Can you work these out from the model? Positions are in its coordinate system, mm. Face numbers are marked on the shaded views. A direction names the side the tool comes from. Give positions to 0.01 mm unless a question says otherwise; leave off trailing zeros. Write each loop counter-clockwise with the first axis right and the second up, starting at its lowest first coordinate (ties: lowest second). Pieces come first, ordered by that corner, then holes.
```python
from build123d import *

# Parameters (mm, degrees)
SALIENTE_EXTRUIR1_DEPTH = 16
CROQUIS6_R              = 11.15
CORTAR_EXTRUIR4_DEPTH   = 14
CROQUIS22_R             = 6
CORTAR_EXTRUIR17_DEPTH  = 3
CROQUIS8_R              = 4.05
CORTAR_EXTRUIR6_DEPTH   = 17
CORTAR_EXTRUIR12_DEPTH  = 30
CROQUIS18_R             = 2.675
CORTAR_EXTRUIR13_DEPTH  = 15
CORTAR_EXTRUIR10_DEPTH  = 30
CROQUIS16_R             = 2.675
CORTAR_EXTRUIR11_DEPTH  = 10
CROQUIS19_R             = 2.675
CORTAR_EXTRUIR14_DEPTH  = 17
CORTAR_EXTRUIR19_DEPTH  = 5.5
REDONDEO1_R             = 2


with BuildPart() as part:
    # Croquis2 → Saliente-Extruir1 (new body)
    with BuildSketch(Plane(origin=(0, 0, 0), x_dir=(-1, 0, 0), z_dir=(0, 1, 0))):
        Polygon((0, 0), (-65, 0), (-65, 25), (-35, 25), (-35, 78.5), (0, 78.5), align=None)
    extrude(amount=SALIENTE_EXTRUIR1_DEPTH)

    # Croquis6 → Cortar-Extruir4 (cut)
    with BuildSketch(Plane(origin=(0, 16, 0), x_dir=(-1, 0, 0), z_dir=(0, 1, 0))):
        with Locations((-17.5, 32)):
            Circle(CROQUIS6_R)
    extrude(amount=-CORTAR_EXTRUIR4_DEPTH, mode=Mode.SUBTRACT)

    # Croquis22 → Cortar-Extruir17 (cut, through all)
    with BuildSketch(Plane(origin=(0, 2, 0), x_dir=(1, 0, 0), z_dir=(0, 1, 0))):
        with Locations((17.5, -32)):
            Circle(CROQUIS22_R)
    extrude(amount=-CORTAR_EXTRUIR17_DEPTH, mode=Mode.SUBTRACT)

    # Croquis8 → Cortar-Extruir6 (cut, through all)
    with BuildSketch(Plane(origin=(0, 16, 0), x_dir=(-1, 0, 0), z_dir=(0, 1, 0))):
        with Locations((-17.5, 10)):
            Circle(CROQUIS8_R)
    extrude(amount=-CORTAR_EXTRUIR6_DEPTH, mode=Mode.SUBTRACT)

    # Croquis17 → Cortar-Extruir12 (cut)
    with BuildSketch(Plane(origin=(65, 0, 0), x_dir=(0, 0, -1), z_dir=(1, 0, 0))):
        Polygon((-16.1, 0), (-16.1, 1.5), (-1.5, 1.5), (-1.5, 16.1), (0, 16.1), (0, 0), align=None)
    extrude(amount=-CORTAR_EXTRUIR12_DEPTH, mode=Mode.SUBTRACT)

    # Croquis18 → Cortar-Extruir13 (cut)
    with BuildSketch(Plane(origin=(0, 0, 1.5), x_dir=(-1, 0, 0), z_dir=(0, 0, -1))):
        with Locations((-42.5, 8.75)):
            Circle(CROQUIS18_R)
        with Locations((-57.5, 8.75)):
            Circle(CROQUIS18_R)
    extrude(amount=-CORTAR_EXTRUIR13_DEPTH, mode=Mode.SUBTRACT)

    # Croquis15 → Cortar-Extruir10 (cut)
    with BuildSketch(Plane.XY.offset(78.5)):
        Polygon((0, 0), (0, 16.1), (1.5, 16.1), (1.5, 1.5), (16.1, 1.5), (16.1, 0), align=None)
    extrude(amount=-CORTAR_EXTRUIR10_DEPTH, mode=Mode.SUBTRACT)

    # Croquis16 → Cortar-Extruir11 (cut)
    with BuildSketch(Plane.ZY.offset(-1.5)):
        with Locations((56, 8.75)):
            Circle(CROQUIS16_R)
        with Locations((71, 8.75)):
            Circle(CROQUIS16_R)
    extrude(amount=-CORTAR_EXTRUIR11_DEPTH, mode=Mode.SUBTRACT)

    # Croquis19 → Cortar-Extruir14 (cut, through all)
    with BuildSketch(Plane(origin=(0, 16, 0), x_dir=(1, 0, 0), z_dir=(0, 1, 0))):
        with Locations((6.580936897, -6.580936897)):
            Circle(CROQUIS19_R)
        with Locations((25.84554815, -69.34554815)):
            Circle(CROQUIS19_R)
    extrude(amount=-CORTAR_EXTRUIR14_DEPTH, mode=Mode.SUBTRACT)

    # Croquis23 → Cortar-Extruir19 (cut)
    with BuildSketch(Plane(origin=(0, 16, 0), x_dir=(1, 0, 0), z_dir=(0, 1, 0))):
        with BuildLine():
            Line((35, -78.5), (7.5, -78.5))
            Line((7.5, -78.5), (7.5, -27.068215333))
            ThreePointArc((7.5, -27.068215333), (11.612169289, -22.531317435), (17.5, -20.85))
            Line((17.5, -20.85), (65, -20.85))
            Line((65, -20.85), (65, -25))
            Line((65, -25), (35, -25))
            Line((35, -25), (35, -78.5))
        make_face()
    extrude(amount=-CORTAR_EXTRUIR19_DEPTH, mode=Mode.SUBTRACT)

    # Redondeo1
    redondeo1_edges = [part.edges().sort_by_distance(p)[0] for p in [
        (50, 1.5, 1.5),
        (1.5, 1.5, 63.5),
    ]]
    fillet(redondeo1_edges, radius=REDONDEO1_R)


solid = part.part
```
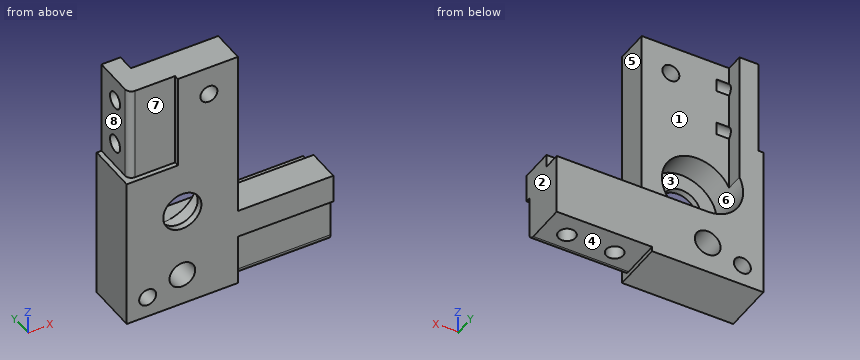
1) Suppose I cut it at C-C on y = 7. State how many separate pieces and enclosed holes the cut face has, plus the area to 3 significant figures.
Values follow:
separate pieces: 1
enclosed holes: 4
area: 2,720 mm2
2) Suppose I cut it at A-A on z = 63.5. Write out the boundary of the cut face in (x, y), plus the area to 3 significant figures.
Values follow:
outline: (1.5, 3.5) arc R2 ccw to (3.5, 1.5) - (16.1, 1.5) - (16.1, 0) - (35, 0) - (35, 10.5) - (7.5, 10.5) - (7.5, 16) - (1.5, 16) - close
area: 362 mm2
3) Suppose I cut it at D-D on z = 7.5. Write out the boundary of the cut face in (x, y) (3 decimals), plus the area to 3 significant figures.
Values follow:
outline: (0, 0) - (4.069, 0) - (4.069, 16) - (0, 16) - close; (9.093, 0) - (14.314, 0) - (14.314, 16) - (9.093, 16) - close; (20.686, 0) - (35, 0) - (35, 1.5) - (65, 1.5) - (65, 16) - (20.686, 16) - close; hole circle Ø5.35 at (42.5, 8.75); hole circle Ø5.35 at (57.5, 8.75)
area: 768 mm2
4) Suppose I cut it at B-B on x = 46.5. Write out the boundary of the cut face in (y, z).
Values follow:
outline: (0, 16.1) - (1.5, 16.1) - (1.5, 3.5) arc R2 ccw to (3.5, 1.5) - (16, 1.5) - (16, 20.85) - (10.5, 20.85) - (10.5, 25) - (0, 25) - close
5) For the marked faces 4, 5, 6, 7 and 8, which set-ups out of +Z, -Z, +X, -X, +Y, -Y let a thin tool reach every point of the face, with its end or its side?
Values follow:
face 4: -Z, +X, +Y, -Y
face 5: +Z, +X, +Y, -Y
face 6: +Y
face 7: +Z, -X, -Y
face 8: +Z, -X, +Y, -Y
6) Please list where these lines run through material, in increasing order: L1, parallel to Z at x = 26, y = 1.5; L2, parallel to Z at x = 37.5, y = 12.25; L3, parallel to Y at x = 56.5, z = 24.
Values follow:
L1: z = 0 to 66.68, 72.02 to 78.5
L2: z = 1.5 to 20.85
L3: y = 0 to 10.5
7) For pin 1 Ø4 at (y, z) = (13.5, 31) entering from +X; pin 2 Ø6 at (x, y) = (43, 8.5) entering from -Z; pin 3 Ø5 at (y, z) = (7.5, 71) entering from -X, each with a flat end and sliding along its axis, tell me the tip position at first contact or that it passes through.
Values follow:
pin 1: stops at x = 6.76
pin 2: stops at z = 1.5
pin 3: stops at x = 1.5
8) If we mould it in two halves opening along X, with no side actions, what happens to the marked faces 1, 2 and 3? For each: +X half, -X half, draft (parallel to the pull), parting line (faces both ways), or undercut.
Values follow:
face 1: draft
face 2: +X half
face 3: undercut
